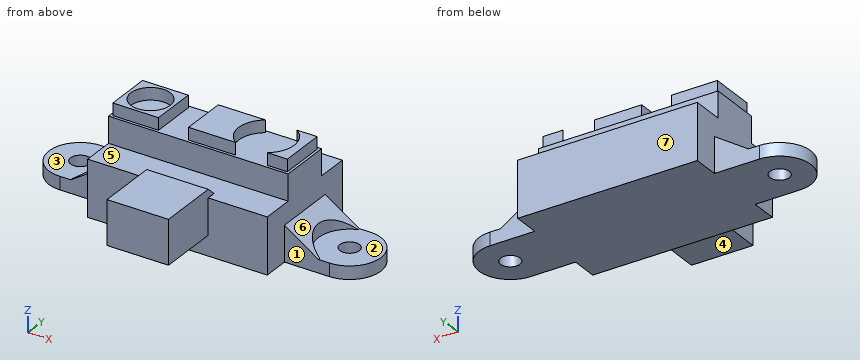
from build123d import *

# Parameters (mm, degrees)
SKETCH1_R           = 1.6
BOSS_EXTRUDE1_DEPTH = 13.5
CUT_EXTRUDE2_DEPTH  = 54.452572483
SKETCH3_W           = 4.3
SKETCH3_H           = 5.25
CUT_EXTRUDE4_DEPTH  = 54.452572483
SKETCH4_W           = 7.5
SKETCH4_H           = 7.5
SKETCH4_R           = 3.233378309
BOSS_EXTRUDE2_DEPTH = 2
CUT_EXTRUDE6_START  = -7.05
SKETCH5_R           = 5.136449747
CUT_EXTRUDE6_DEPTH  = 7.05
SKETCH6_W           = 10.1
SKETCH6_H           = 7.260831794
BOSS_EXTRUDE3_DEPTH = 10
BOSS_EXTRUDE4_DEPTH = 10.1


with BuildPart() as part:
    # Sketch1 → Boss-Extrude1 (new body)
    with BuildSketch(Plane.XY):
        with BuildLine():
            Line((6.026068185, 19.19002712), (35.526068185, 19.19002712))
            Line((35.526068185, 19.19002712), (35.526068185, 14.876476867))
            Line((35.526068185, 14.876476867), (42.891358492, 14.876476867))
            ThreePointArc((42.891358492, 14.876476867), (48.027808239, 9.74002712), (42.891358492, 4.603577373))
            Line((42.891358492, 4.603577373), (35.526068185, 4.603577373))
            Line((35.526068185, 4.603577373), (35.526068185, 0.29002712))
            Line((35.526068185, 0.29002712), (6.026068185, 0.29002712))
            Line((6.026068185, 0.29002712), (6.026068185, 4.603577373))
            Line((6.026068185, 4.603577373), (-1.339222121, 4.603577373))
            ThreePointArc((-1.339222121, 4.603577373), (-6.475671868, 9.74002712), (-1.339222121, 14.876476867))
            Line((-1.339222121, 14.876476867), (6.026068185, 14.876476867))
            Line((6.026068185, 14.876476867), (6.026068185, 19.19002712))
        make_face()
        with Locations((-1.339222121, 9.74002712)):
            Circle(SKETCH1_R, mode=Mode.SUBTRACT)
        with Locations((42.891358492, 9.74002712)):
            Circle(SKETCH1_R, mode=Mode.SUBTRACT)
    extrude(amount=BOSS_EXTRUDE1_DEPTH)

    # Sketch2 → Cut-Extrude2 (cut, through all)
    with BuildSketch(Plane(origin=(0, 0, 0), x_dir=(1, 0, 0), z_dir=(0, 1, 0))):
        Polygon((-6.475671868, -2.15), (-6.475671868, 0), (-10.044911126, 0), (-10.044911126, -17.049735049), (6.026068185, -17.049735049), (6.026068185, -5.837365249), (0.437350873, -2.15), align=None)
        Polygon((48.027808239, 0), (51.597047497, 0), (51.597047497, -17.049735049), (35.526068185, -17.049735049), (35.526068185, -5.837365249), (41.114785497, -2.15), (48.027808239, -2.15), align=None)
    extrude(amount=CUT_EXTRUDE2_DEPTH, mode=Mode.SUBTRACT)

    # Sketch3 → Cut-Extrude4 (cut, through all)
    with BuildSketch(Plane(origin=(0, 0, 0), x_dir=(0, 0, -1), z_dir=(1, 0, 0))):
        with Locations((-11.35, 16.56502712)):
            Rectangle(SKETCH3_W, SKETCH3_H)
        with Locations((-11.35, 2.91502712)):
            Rectangle(SKETCH3_W, SKETCH3_H)
    extrude(amount=CUT_EXTRUDE4_DEPTH, mode=Mode.SUBTRACT)

    # Sketch4 → Boss-Extrude2 (add)
    # profile 1 of 3: a face of its own
    with BuildSketch(Plane.XY.offset(13.5)):
        with Locations((10.1915125, 9.743497044)):
            Rectangle(SKETCH4_W, SKETCH4_H)
        with Locations((10.1915125, 9.743497044)):
            Circle(SKETCH4_R, mode=Mode.SUBTRACT)
    # profile 2 of 3: a face of its own
    with BuildSketch(Plane.XY.offset(13.5)):
        with BuildLine():
            Line((35.102590636, 13.493497044), (31.813216882, 13.493497044))
            ThreePointArc((31.813216882, 13.493497044), (33.77792813, 9.743497044), (31.813216882, 5.993497044))
            Line((31.813216882, 5.993497044), (35.102590636, 5.993497044))
            Line((35.102590636, 5.993497044), (35.102590636, 13.493497044))
        make_face()
    # profile 3 of 3: a face of its own
    with BuildSketch(Plane.XY.offset(13.5)):
        with BuildLine():
            Line((18.865933267, 13.493497044), (18.865933267, 5.993497044))
            Line((18.865933267, 5.993497044), (26.620387797, 5.993497044))
            ThreePointArc((26.620387797, 5.993497044), (24.655676549, 9.743497044), (26.620387797, 13.493497044))
            Line((26.620387797, 13.493497044), (18.865933267, 13.493497044))
        make_face()
    extrude(amount=BOSS_EXTRUDE2_DEPTH)

    # Sketch5 → Cut-Extrude6 (cut)
    with BuildSketch(Plane.XY.offset(9.2).offset(CUT_EXTRUDE6_START)):
        with Locations((-1.339222121, 9.74002712)):
            Circle(SKETCH5_R)
        with Locations((42.891358492, 9.74002712)):
            Circle(SKETCH5_R)
    extrude(amount=CUT_EXTRUDE6_DEPTH, mode=Mode.SUBTRACT)

    # Sketch6 → Boss-Extrude3 (add)
    with BuildSketch(Plane.XZ.offset(-0.29002712)):
        with Locations((20.776068185, 6.930415897)):
            Rectangle(SKETCH6_W, SKETCH6_H)
    extrude(amount=BOSS_EXTRUDE3_DEPTH)

    # Sketch7 → Boss-Extrude4 (add)
    with BuildSketch(Plane(origin=(25.826068185, 0, 0), x_dir=(0, 0, -1), z_dir=(1, 0, 0))):
        Polygon((-10.560831794, 0.29002712), (-9.2, 0.29002712), (-9.2, 1.787728589), align=None)
    extrude(amount=-BOSS_EXTRUDE4_DEPTH)


solid = part.part
Geometry check sheet. Reference: the model listing, model coordinates, mm. Face numbers are marked on the shaded views. A direction names the side the tool comes from. Coordinates: 2 decimals unless noted, no trailing zeros. Order: outer loops, then holes, each group sorted by start corner. A loop starts at its lowest first (then second) coordinate and runs counter-clockwise, first axis right, second up. Notation, with made-up numbers: (64, 76) - (106, 76) arc R27 cw to (106, 97) - close; hole circle Ø6 at (29, -2.75). An arc over 180 degrees is marked (long way). Answer in a Markdown table with one row per item. Add a question column.
1) Material ranges on line 1 along X through (y, z) = (-4.75, 9.5); line 2 along X through (y, z) = (7, 6); line 3 along Y through (x, z) = (25, 3), recorded low to high. Write a range as [from, to].
2) Cross-section at C-C, the plane x = 10. Record the cut outline in (y, z).
3) Cross-section at D-D, the plane z = 12.5. Record the cut outline in (x, y).
4) Cross-section at B-B, the plane y = 1. Record the cut outline in (x, z).
5) Gauge pin test, flat ends, axial feed: P1, Ø1.6, axis at x = 23.5, z = 15, coming from the -Y side; P2, Ø3, axis at x = -1.34, y = 9.74, coming from the -Z side; P3, Ø4, axis at x = 10.19, y = 9.74, coming from the +Z side; P4, Ø1, axis at y = 11, z = 14.5, coming from the +X side. Record the tip position at first contact, or that the pin passes through.
6) Set-up check for the marked faces 1, 2, 3 and 4: record each of +Z, -Z, +X, -X, +Y, -Y from which the full face is reachable in a straight line by a thin tool's end or side.
7) Cross-section at A-A, the plane z = 7.75. Record the cut outline in (x, y).
8) Release check for a two-part mould opening along Y. For the marked faces 5, 6 and 7 record: +Y half, -Y half, draft (parallel to the pull), parting line (faces both ways), or undercut.
Check result:
| question | item | result |
|---|---|---|
| 1 | line 1 | x = [15.73, 25.83] |
| 1 | line 2 | x = [6.03, 35.53] |
| 1 | line 3 | y = [0.29, 19.19] |
| 2 | outline | (0.29, 0) - (19.19, 0) - (19.19, 9.2) - (13.94, 9.2) - (13.94, 13.5) - (13.49, 13.5) - (13.49, 15.5) - (12.97, 15.5) - (12.97, 13.5) - (6.52, 13.5) - (6.52, 15.5) - (5.99, 15.5) - (5.99, 13.5) - (5.54, 13.5) - (5.54, 9.2) - (0.29, 9.2) - close |
| 3 | outline | (6.03, 5.54) - (35.53, 5.54) - (35.53, 13.94) - (6.03, 13.94) - close |
| 4 | outline | (6.03, 0) - (35.53, 0) - (35.53, 9.2) - (25.83, 9.2) - (25.83, 9.92) - (15.73, 9.92) - (15.73, 9.2) - (6.03, 9.2) - close |
| 5 | P1 | stops at y = 5.99 |
| 5 | P2 | passes through |
| 5 | P3 | stops at z = 13.5 |
| 5 | P4 | stops at x = 35.1 |
| 6 | face 1 | +Z, -Z, +X, -Y |
| 6 | face 2 | +Z, +X |
| 6 | face 3 | +Z, -X |
| 6 | face 4 | -Z, +X, -X, -Y |
| 7 | outline | (6.03, 0.29) - (15.73, 0.29) - (15.73, -9.71) - (25.83, -9.71) - (25.83, 0.29) - (35.53, 0.29) - (35.53, 19.19) - (6.03, 19.19) - close |
| 8 | face 5 | undercut |
| 8 | face 6 | draft |
| 8 | face 7 | +Y half |
